Design review of the part shown in the three views and the two pictorial views. Dimensions are in mm from the part's minimum x, y and z. A direction names the side the tool comes from. Give positions to 0.01 mm unless a question says otherwise; leave off trailing zeros. Loops run counter-clockwise (first coordinate to the right, second up) from the corner with the lowest first, then second, coordinate; pieces in that order, holes last. Notation, with made-up numbers: (37, 65.25) - (56, 65.25) arc R30 cw to (56, 93.25) - close; hole circle Ø11 at (66.25, 68). An arc over 180 degrees is marked (long way). Use CSV: the item, a comma, the result in double quotes. Start each with the question number.
1. Mouldability with a two-part tool opening along Z and no side actions: class the marked faces 3, 4 and 5 as pulls with the +Z half, pulls with the -Z half, needs draft (parallel to the pull), parting line crosses it, or undercut.
2. Take a section at A-A on y = 5. Give the boundary of the cut face in (x, z).
3. Take a section at D-D on y = 13.25. Give the boundary of the cut face in (x, z).
4. For pin 1 (3 mm diameter, centred on x = 4.5, z = 2.5, fed in from -Y), flat-tipped, find the tip position at first contact; note if it passes through.
5. Take a section at B-B on x = 5.75. Give the boundary of the cut face in (y, z).
6. For the marked faces 1 and 2, list the 3-axis set-ups (+Z, -Z, +X, -X, +Y, -Y) from which the entire face can be reached by the end or side of a thin tool; tool diameter is ignored.
7. Wall thickness on line 1 (Z direction, x = 6, y = 5); line 2 (X direction, y = 16, z = 5.25); line 3 (X direction, y = 8.5, z = 4.5): over which ranges is each line inside the solid? List them lowest first.
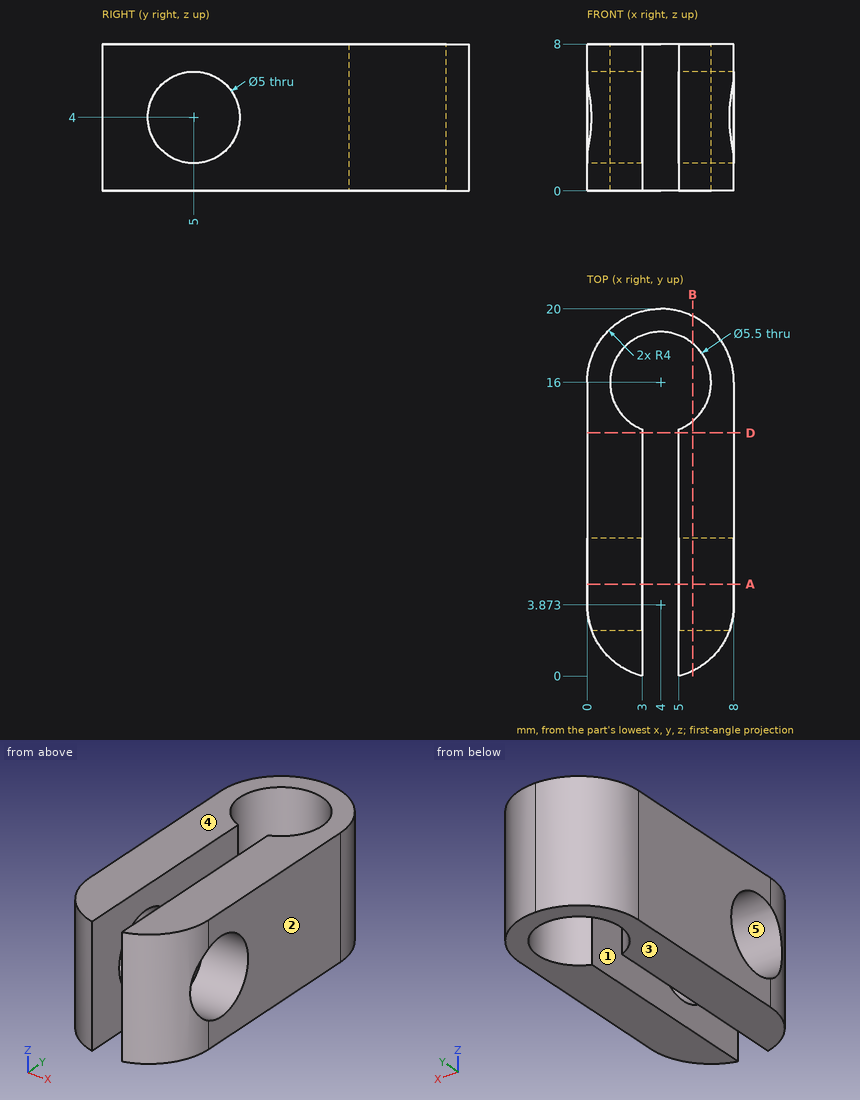
Check result:
1,face 3,"pulls with the -Z half"
1,face 4,"pulls with the +Z half"
1,face 5,"undercut"
2,outline,"(0, 0) - (3, 0) - (3, 1.5) - (0, 1.5) - close; (0, 6.5) - (3, 6.5) - (3, 8) - (0, 8) - close; (5, 0) - (8, 0) - (8, 1.5) - (5, 1.5) - close; (5, 6.5) - (8, 6.5) - (8, 8) - (5, 8) - close"
3,outline,"(0, 0) - (3, 0) - (3, 8) - (0, 8) - close; (5, 0) - (8, 0) - (8, 8) - (5, 8) - close"
4,pin 1,"stops at y = 0"
5,outline,"(0.28, 0) - (13.88, 0) - (13.88, 8) - (0.28, 8) - close; (18.12, 0) - (19.6, 0) - (19.6, 8) - (18.12, 8) - close; hole circle Ø5 at (5, 4)"
6,face 1,"+Z, -Z, -Y"
6,face 2,"+Z, -Z, +X, +Y, -Y"
7,line 1,"z = 0 to 1.5, 6.5 to 8"
7,line 2,"x = 0 to 1.25, 6.75 to 8"
7,line 3,"x = 0 to 3, 5 to 8"
